For this review, use the dimensioned drawing (mm, ordinates from the lowest corner) and the shaded views. Coordinates: 2 decimals unless noted, no trailing zeros. Order: outer loops, then holes, each group sorted by start corner. A loop starts at its lowest first (then second) coordinate and runs counter-clockwise, first axis right, second up. Notation, with made-up numbers: M -2,-35.5 L 35,-35.5 A16 cw 35,-22.5 Z; hole C 37.5,15.5 d1. An arc over 180 degrees is marked long. Answer in a Markdown table with one row per item.
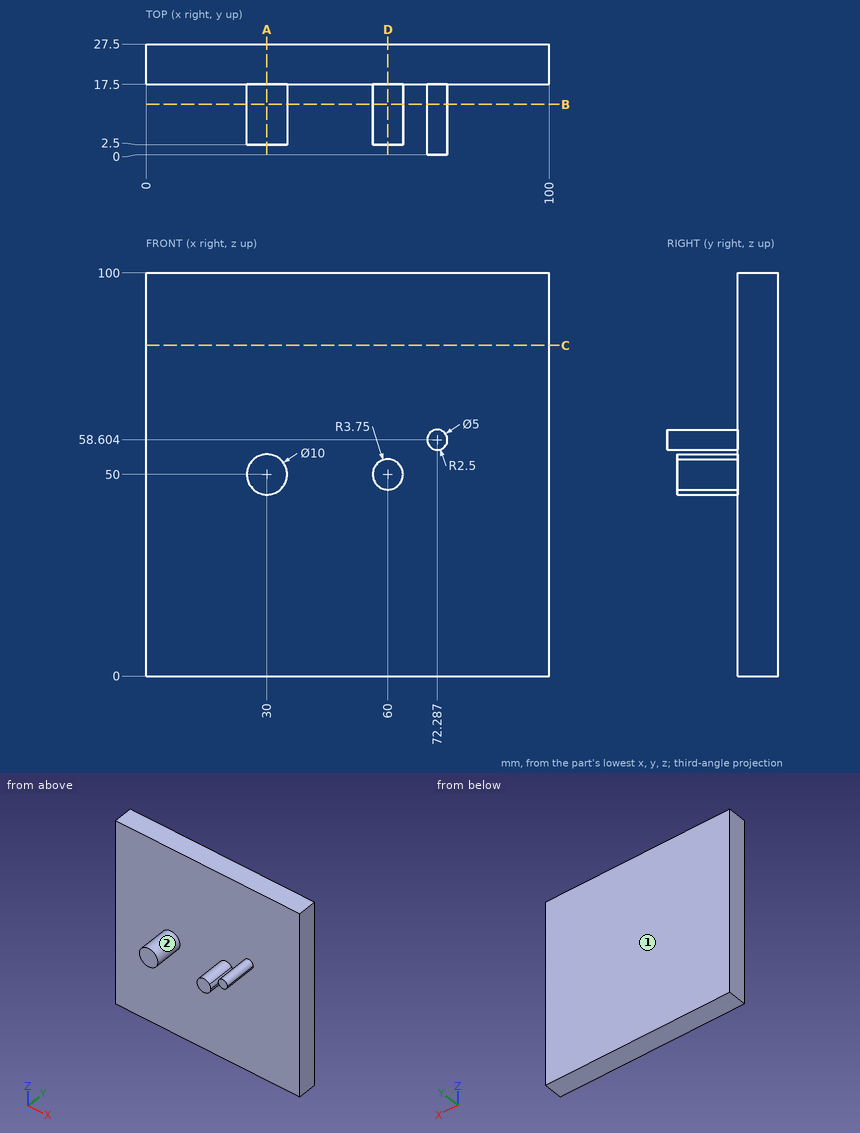
(1) Draft analysis for pull direction X (two halves, no side actions). For the marked faces 1 and 2, state which applies: pulls with the +X half, pulls with the -X half, needs draft (parallel to the pull), parting line crosses it, or undercut.
Return value:
| item | result |
|---|---|
| face 1 | needs draft |
| face 2 | undercut |
(2) Add section A-A, the plane x = 30. Give the boundary of the cut face in (y, z).
Return value:
| item | result |
|---|---|
| outline | M 2.5,45 L 17.5,45 L 17.5,0 L 27.5,0 L 27.5,100 L 17.5,100 L 17.5,55 L 2.5,55 Z |
(3) Insertion check: pin 1 Ø10 at (x, y) = (29, 19) entering from -Z; pin 2 Ø6 at (x, z) = (82.5, 61.5) entering from -Y; pin 3 Ø12 at (y, z) = (6, 44) entering from +X; pin 4 Ø11 at (x, z) = (28, 52) entering from -Y. Each pin has a flat end and moves straight along its axis. Give the tip position at first contact, or say it passes through.
Return value:
| item | result |
|---|---|
| pin 1 | stops at z = 0 |
| pin 2 | stops at y = 17.5 |
| pin 3 | stops at x = 63.75 |
| pin 4 | stops at y = 2.5 |
(4) For line 1 along Y through (x, z) = (7, 26.5); line 2 along Z through (x, y) = (30, 15.25); line 3 along Z through (x, y) = (32, 5.5), list the stretches that pass through material, from the lowest coordinate up. Write a range as from..to.
Return value:
| item | result |
|---|---|
| line 1 | y = 17.5..27.5 |
| line 2 | z = 45..55 |
| line 3 | z = 45.42..54.58 |
(5) Add section C-C, the plane z = 82. Give the boundary of the cut face in (x, y), and give its area (3 significant figures).
Return value:
| item | result |
|---|---|
| outline | M 0,17.5 L 100,17.5 L 100,27.5 L 0,27.5 Z |
| area | 1,000 mm2 |
(6) Add section B-B, the plane y = 12.5. Give the boundary of the cut face in (x, z).
Return value:
| item | result |
|---|---|
| outline | C 30,50 d10; M 63.07,52.15 A3.75 ccw long 63.75,50 A3.75 ccw Z; C 72.29,58.6 d5 |
(7) Add section D-D, the plane x = 60. Give the boundary of the cut face in (y, z).
Return value:
| item | result |
|---|---|
| outline | M 2.5,46.25 L 17.5,46.25 L 17.5,0 L 27.5,0 L 27.5,100 L 17.5,100 L 17.5,53.75 L 2.5,53.75 Z |
